Geometry check sheet. Reference: the model listing, model coordinates, mm. A direction names the side the tool comes from. Coordinates: 2 decimals unless noted, no trailing zeros. Order: outer loops, then holes, each group sorted by start corner. A loop starts at its lowest first (then second) coordinate and runs counter-clockwise, first axis right, second up. Notation, with made-up numbers: (66.25, 64.5) - (99.25, 64.5) arc R13 cw to (99.25, 81.5) - close; hole circle Ø6 at (-23.5, 22.5). An arc over 180 degrees is marked (long way). Put each result on its own line as item: value.
from build123d import *

# Parameters (mm, degrees)
SKETCH1_W                      = 44.45
SKETCH1_H                      = 76.2
EXTRUDE1_DEPTH                 = 19.05
F_1_4_CLEARANCE_HOLE1_D        = 7.14248
CBORE_FOR_1_4_DOWEL_AT_2_COUNT = 2
CBORE_FOR_1_4_DOWEL_AT_2_PITCH = 19.05
F_3_16_0_1875_DIAMETER_HOLE1_D = 4.7625


with BuildPart() as part:
    # Sketch1 → Extrude1 (new body)
    with BuildSketch(Plane.XY):
        Rectangle(SKETCH1_W, SKETCH1_H)
    extrude(amount=EXTRUDE1_DEPTH)

    # 1/4 Clearance Hole1 (through all)
    with Locations(Plane(origin=(22.225, 0, 0), x_dir=(0, 0, -1), z_dir=(1, 0, 0))):
        with Locations((-9.525, 25.4), (-9.525, -25.4)):
            Hole(F_1_4_CLEARANCE_HOLE1_D / 2)

    # Sketch4 → CBORE for 1/4 DOWEL (revolve, cut)
    with BuildSketch(Plane(origin=(22.225, -9.525, 9.525), x_dir=(0, 0, -1), z_dir=(0, 1, 0))):
        Polygon((0, 0), (0, 11.559732465), (3.175, 9.652), (3.175, 2.54), (3.1877, 2.54), (3.1877, 0.3683), (3.556, 0), align=None)
    cbore_for_1_4_dowel = revolve(axis=Axis((28.575, -9.525, 9.525), (-1, 0, 0)), mode=Mode.SUBTRACT)

    # CBORE for 1/4 DOWEL at 2: CBORE for 1/4 DOWEL ×2
    with Locations(*[(0, i * CBORE_FOR_1_4_DOWEL_AT_2_PITCH, 0) for i in range(1, CBORE_FOR_1_4_DOWEL_AT_2_COUNT)]):
        add(cbore_for_1_4_dowel, mode=Mode.SUBTRACT)

    # 3/16 (0.1875) Diameter Hole1 (through all)
    with Locations(Plane(origin=(22.225, 0, 0), x_dir=(0, 0, -1), z_dir=(1, 0, 0))):
        with Locations((-9.525, 9.525), (-9.525, -9.525)):
            Hole(F_3_16_0_1875_DIAMETER_HOLE1_D / 2)

    # Mirror1: CBORE for 1/4 DOWEL across plane
    add(cbore_for_1_4_dowel.mirror(Plane(origin=(0, 0, 0), x_dir=(0, 0, 1), z_dir=(1, 0, 0))), mode=Mode.SUBTRACT)

    # Mirror1 copy 1 sketch → Mirror1 copy 1 (revolve, cut)
    with BuildSketch(Plane(origin=(-22.225, 9.525, 9.525), x_dir=(0, 0, -1), z_dir=(0, 1, 0))):
        Polygon((0, 0), (0, -11.559732465), (3.175, -9.652), (3.175, -2.54), (3.1877, -2.54), (3.1877, -0.3683), (3.556, 0), align=None)
    revolve(axis=Axis((-28.575, 9.525, 9.525), (-1, 0, 0)), mode=Mode.SUBTRACT)


solid = part.part
Q1. Section check A-A on y = 25.4. Record the boundary of the cut face in (x, z) (3 decimals).
Answer block:
outline: (-22.225, 0) - (22.225, 0) - (22.225, 5.954) - (-22.225, 5.954) - close; (-22.225, 13.096) - (22.225, 13.096) - (22.225, 19.05) - (-22.225, 19.05) - close
Q2. Section check B-B on x = 13.5. Record the boundary of the cut face in (y, z) (3 decimals), then the cut area to 3 significant figures.
Answer block:
outline: (-38.1, 0) - (38.1, 0) - (38.1, 19.05) - (-38.1, 19.05) - close; hole circle Ø7.142 at (-25.4, 9.525); hole circle Ø6.35 at (-9.525, 9.525); hole circle Ø6.35 at (9.525, 9.525); hole circle Ø7.142 at (25.4, 9.525)
area: 1,310 mm^2
Q3. Section check C-C on z = 9.25. State how many separate pieces and enclosed holes the cut face has, then the cut area to 3 significant figures.
Answer block:
separate pieces: 5
enclosed holes: 0
area: 2,270 mm^2
Q4. Depth check by flat-ended pin: pin 1 Ø6 at (y, z) = (9.525, 9.525) entering from +X; pin 2 Ø5 at (y, z) = (9.525, 9.525) entering from -X; pin 3 Ø4 at (y, z) = (-9.525, 9.525) entering from +X. Enter the tip coordinate at first touch or a pass-through.
Answer block:
pin 1: stops at x = 12.47
pin 2: stops at x = -12.17
pin 3: passes through
Q5. Access from +Z, -Z, +X, -X, +Y, -Y to the whole of each face (thin tool, end or side, straight path). Record for faces 4 (the cylindrical face through (-0.311, 21.914, 8.751)), 5 (the cylindrical face through (16.18, 11.46, 12.04)), 6 (the cylindrical face through (-16.18, 11.46, 12.04)).
Answer block:
face 4: +X, -X
face 5: +X
face 6: -X
Q6. Thickness scan on L1, parallel to Y at x = -15, z = 9.75; L2, parallel to Y at x = -3, z = 10.75; L3, parallel to Y at x = 3.5, z = 12. Record the ranges inside material, lowest first. Write a range as [from, to].
Answer block:
L1: y = [-38.1, -28.96], [-21.84, -12.69], [-6.36, 6.36], [12.69, 21.84], [28.96, 38.1]
L2: y = [-38.1, -28.75], [-22.05, -11.57], [-7.48, 7.48], [11.57, 22.05], [28.75, 38.1]
L3: y = [-38.1, -27.97], [-22.83, 22.83], [27.97, 38.1]
Q7. Draft check along Z on faces 1 (the flat face through (0, 38.1, 9)), 2 (the cylindrical face through (-20.786, -11.679, 11.874)), 3 (the flat face through (0, 1, 19.05)). Enter one of: pulls with the +Z half, pulls with the -Z half, needs draft (parallel to the pull), parting line crosses it, or undercut.
Answer block:
face 1: needs draft
face 2: undercut
face 3: pulls with the +Z half
